Model file for the job. Use its own axes, mm. Coordinates: 2 decimals unless noted, no trailing zeros. Write each loop counter-clockwise with the first axis right and the second up, starting at its lowest first coordinate (ties: lowest second). Pieces come first, ordered by that corner, then holes. Notation, with made-up numbers: (40.25, -24.5) - (91.25, -24.5) arc R21 ccw to (91.25, -3.5) - close; hole circle Ø9 at (58.5, 61). An arc over 180 degrees is marked (long way). Put each result on its own line as item: value. Start each with the question number.
1. Drop flat-ended pins along their axis: P1, Ø3, axis at x = -21.52, z = 31.64, coming from the +Y side; P2, Ø1, axis at x = 26.5, y = -1, coming from the +Z side. Give the stop position or say it passes through.
2. Pull direction X, two halves, no side cores. Call faces 1 (the face through (-23.927, -1.207, -6.359)), 2 (the face through (-21, -1, 37.985)), 3 (the face through (41.984, -1, -26)): released by +X, released by -X, zero draft, split by the parting line, or undercut.
3. Saw through at C-C, the plane z = 17. Write the cut outline in (x, y).
4. Drill centre lines: L1, parallel to Z at x = -21.5, y = -0.4; L2, parallel to Z at x = -19.5, y = -2; L3, parallel to X at y = -2.2, z = 30. Where is each one in solid material? Low to high. Write a range as from..to.
5. Saw through at A-A, the plane x = 3. Write the cut outline in (y, z), plus the area to 3 significant figures.
6. Saw through at B-B, the plane y = -1. Write the cut outline in (x, z), plus the area to 3 significant figures.
7. Saw through at D-D, the plane x = 33.5. Write the cut outline in (y, z), plus the area to 3 significant figures.
```python
from build123d import *

# Parameters (mm, degrees)
F1_DEPTH = 2.38125
F2_R     = 0.508
F3_R     = 2.413
F4_DEPTH = 2.38125


with BuildPart() as f1:
    # F0 (on Front) → F1 (new body)
    with BuildSketch(Plane.XZ):
        Polygon((-8.816487, 37.985209), (-34.216487, 37.985209), (-34.216487, -38.214791), (41.983513, -38.214791), (41.983513, -12.814791), align=None)
    extrude(amount=F1_DEPTH)

    # F2
    f2_edges = [f1.edges().sort_by_distance(p)[0] for p in [
        (-34.216487, -1.190625, 37.985209),
        (-8.816487, -1.190625, 37.985209),
        (-34.216487, -1.190625, -38.214791),
        (41.983513, -1.190625, -12.814791),
        (41.983513, -1.190625, -38.214791),
    ]]
    fillet(f2_edges, radius=F2_R)

    # F3 (on face) → F4 (cut)
    with BuildSketch(Plane.XZ.offset(2.38125)):
        with Locations((-21.516487, 31.635209)):
            Circle(F3_R)
        with Locations((-21.516487, 12.585209)):
            Circle(F3_R)
        with Locations((-21.516487, -6.464791)):
            Circle(F3_R)
        with Locations((-21.516487, -25.514791)):
            Circle(F3_R)
        with Locations((3.883513, -25.514791)):
            Circle(F3_R)
        with Locations((29.283513, -25.514791)):
            Circle(F3_R)
    extrude(amount=-F4_DEPTH, mode=Mode.SUBTRACT)


solid = f1.part
```
Final values:
1. P1: passes through
1. P2: stops at z = 3.17
2. face 1: undercut
2. face 2: zero draft
2. face 3: released by +X
3. outline: (-34.22, -2.38) - (12.17, -2.38) - (12.17, 0) - (-34.22, 0) - close
4. L1: z = -38.21..-27.93, -23.1..-8.88, -4.05..10.17, 15..29.22, 34.05..37.99
4. L2: z = -38.21..-26.84, -24.19..-7.79, -5.14..11.26, 13.91..30.31, 32.96..37.99
4. L3: x = -34.22..-23.29, -19.74..-0.83
5. outline: (-2.38, -38.21) - (0, -38.21) - (0, -27.76) - (-2.38, -27.76) - close; (-2.38, -23.27) - (0, -23.27) - (0, 26.17) - (-2.38, 26.17) - close
5. area: 143 mm²
6. outline: (-34.22, -37.71) arc R0.51 ccw to (-33.71, -38.21) - (41.48, -38.21) arc R0.51 ccw to (41.98, -37.71) - (41.98, -13.03) arc R0.51 ccw to (41.83, -12.67) - (-8.67, 37.84) arc R0.51 ccw to (-9.03, 37.99) - (-33.71, 37.99) arc R0.51 ccw to (-34.22, 37.48) - close; hole circle Ø4.83 at (-21.52, -25.51); hole circle Ø4.83 at (-21.52, -6.46); hole circle Ø4.83 at (-21.52, 12.59); hole circle Ø4.83 at (-21.52, 31.64); hole circle Ø4.83 at (3.88, -25.51); hole circle Ø4.83 at (29.28, -25.51)
6. area: 4,410 mm²
7. outline: (-2.38, -38.21) - (0, -38.21) - (0, -4.33) - (-2.38, -4.33) - close
7. area: 80.7 mm²
